Autodesk Inventor part; units mm, degrees
ref_plane "YZ Plane" through (0, 0, 0) normal (1, 0, 0) x (0, 1, 0)
ref_plane "XZ Plane" through (0, 0, 0) normal (0, 1, 0) x (-1, 0, 0)
ref_plane "XY Plane" through (0, 0, 0) normal (0, 0, 1) x (1, 0, 0)
sketch "Эскиз1" plane through (0, 0, 0) normal (0, 0, 1) x (1, 0, 0)
  arc A0 (5.088, 16.8311) -> (-4.912, 6.8311) centre (5.088, 6.8311) ccw
  line L0 (7.3397, 7.2282) -> (8.088, 7.2282)
  line L1 (7.3397, 7.2282) -> (9.538, 3.3282)
  line L2 (2.8364, 7.2282) -> (0.638, 3.3282)
  line L3 (7.3397, -0.5718) -> (9.538, 3.3282)
  line L4 (2.8364, -0.5718) -> (0.638, 3.3282)
  line L5 (2.088, 12.1282) -> (8.088, 12.1282)
  line L6 (8.088, 12.1282) -> (8.088, 7.2282)
  line L7 (2.088, 7.2282) -> (2.8364, 7.2282)
  line L8 (2.088, 12.1282) -> (2.088, 7.2282)
  line L9 (-4.912, 6.8311) -> (-4.912, -0.1747)
  arc A1 (-4.912, -0.1747) -> (15.088, -0.1747) centre (5.088, -0.1747) ccw
  line L10 (15.088, -0.1747) -> (15.088, 10.1176)
  line L11 (7.3397, -0.5718) -> (8.088, -0.5718)
  line L12 (2.088, -5.4718) -> (8.088, -5.4718)
  line L13 (8.088, -5.4718) -> (8.088, -0.5718)
  line L14 (2.088, -0.5718) -> (2.8364, -0.5718)
  line L15 (2.088, -5.4718) -> (2.088, -0.5718)
  line L16 (5.088, 16.8311) -> (41.732, 39.3305)
  line L17 (46.9644, 30.8087) -> (16.0416, 11.822)
  arc A2 (48.6091, 37.6858) -> (41.732, 39.3305) centre (44.3482, 35.0696) ccw
  arc A3 (46.9644, 30.8087) -> (48.6091, 37.6858) centre (44.3482, 35.0696) ccw
  arc A4 (16.0416, 11.822) -> (15.088, 10.1176) centre (17.088, 10.1176) ccw
  point P0 (5.088, 3.3282)
  point P1 (15.088, 11.2365)
extrude "Выдавливание1" add sketch "Эскиз1" along normal blind 5
properties part number "В. шарн. - держатель соединителя"
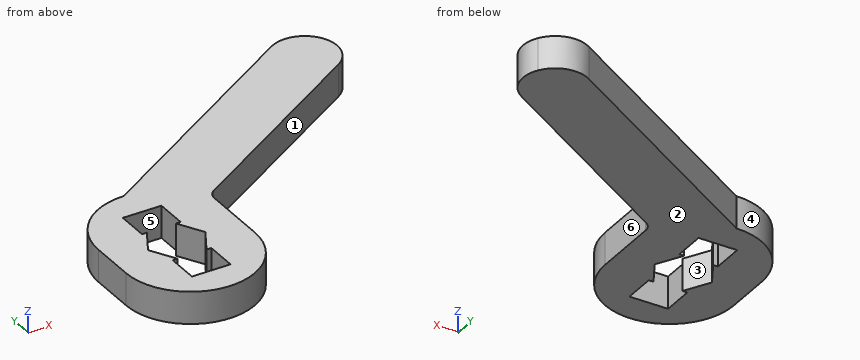
Can you work these out from the model? Positions are in its coordinate system, mm. Face numbers are marked on the shaded views. A direction names the side the tool comes from. Give positions to 0.01 mm unless a question says otherwise; leave off trailing zeros. Order: outer loops, then holes, each group sorted by start corner. A loop starts at its lowest first (then second) coordinate and runs counter-clockwise, first axis right, second up. Notation, with made-up numbers: M 8,-29.5 L 24,-29.5 A16 ccw 24,-14.5 Z; hole C 46.5,36 d11. An arc over 180 degrees is marked long. Use one line per item in the form item = value.
Item 1: If we section it at D-D, the plane x = 34.5: Write out the boundary of the cut face in (y, z).
Values follow:
outline = M 23.16,0 L 34.89,0 L 34.89,5 L 23.16,5 Z
Item 2: If I drill on line 1 along X through (y, z) = (4.5, 3.15); line 2 along X through (y, z) = (6.5, 3.3); line 3 along Y through (x, z) = (1.5, 1.1), over which ranges is the centre line in solid material (lowest first)? Write a range as [from, to].
Values follow:
line_1 = [-4.91, 1.3], [8.88, 15.09]
line_2 = [-4.91, 2.43], [7.75, 15.09]
line_3 = [-9.51, 1.8], [4.86, 16.17]
Item 3: If we section it at C-C, the plane y = 24: Write out the boundary of the cut face in (x, z).
Values follow:
outline = M 16.76,0 L 35.88,0 L 35.88,5 L 16.76,5 Z
Item 4: If we section it at B-B, the plane y = 9: Write out the boundary of the cut face in (x, z).
Values follow:
outline = M -4.67,0 L 2.09,0 L 2.09,5 L -4.67,5 Z; M 8.09,0 L 15.09,0 L 15.09,5 L 8.09,5 Z
Item 5: Will these pins go through, and if not, where does the flat tip stop? pin 1 Ø2 at (y, z) = (23.5, 4.5) entering from -X; pin 2 Ø0.6 at (x, z) = (7.5, 3.5) entering from -Y; pin 3 Ø2.5 at (x, z) = (6.5, 1.5) entering from +Y.
Values follow:
pin_1 = 14.32
pin_2 = -9.95
pin_3 = 18.47
Item 6: Thinking about a two-plate mould opening in Y: for the marked faces 1, 2 and 3, which applies, pulls with the +Y half, pulls with the -Y half, needs draft (parallel to the pull), parting line crosses it, or undercut?
Values follow:
face_1 = pulls with the -Y half
face_2 = needs draft
face_3 = undercut
Item 7: For the marked faces 4, 5 and 6, which set-ups out of +Z, -Z, +X, -X, +Y, -Y let a thin tool reach every point of the face, with its end or its side?
Values follow:
face_4 = +Z, -Z, -X, +Y
face_5 = +Z, -Z
face_6 = +Z, -Z, +X, -Y
Item 8: If we section it at A-A, the plane z = 3.8: Write out the boundary of the cut face in (x, y).
Values follow:
outline = M -4.91,-0.17 A10 ccw 15.09,-0.17 L 15.09,10.12 A2 cw 16.04,11.82 L 46.96,30.81 A5 ccw 41.73,39.33 L 5.09,16.83 A10 ccw -4.91,6.83 Z; hole M 0.64,3.33 L 2.84,-0.57 L 2.09,-0.57 L 2.09,-5.47 L 8.09,-5.47 L 8.09,-0.57 L 7.34,-0.57 L 9.54,3.33 L 7.34,7.23 L 8.09,7.23 L 8.09,12.13 L 2.09,12.13 L 2.09,7.23 L 2.84,7.23 Z
